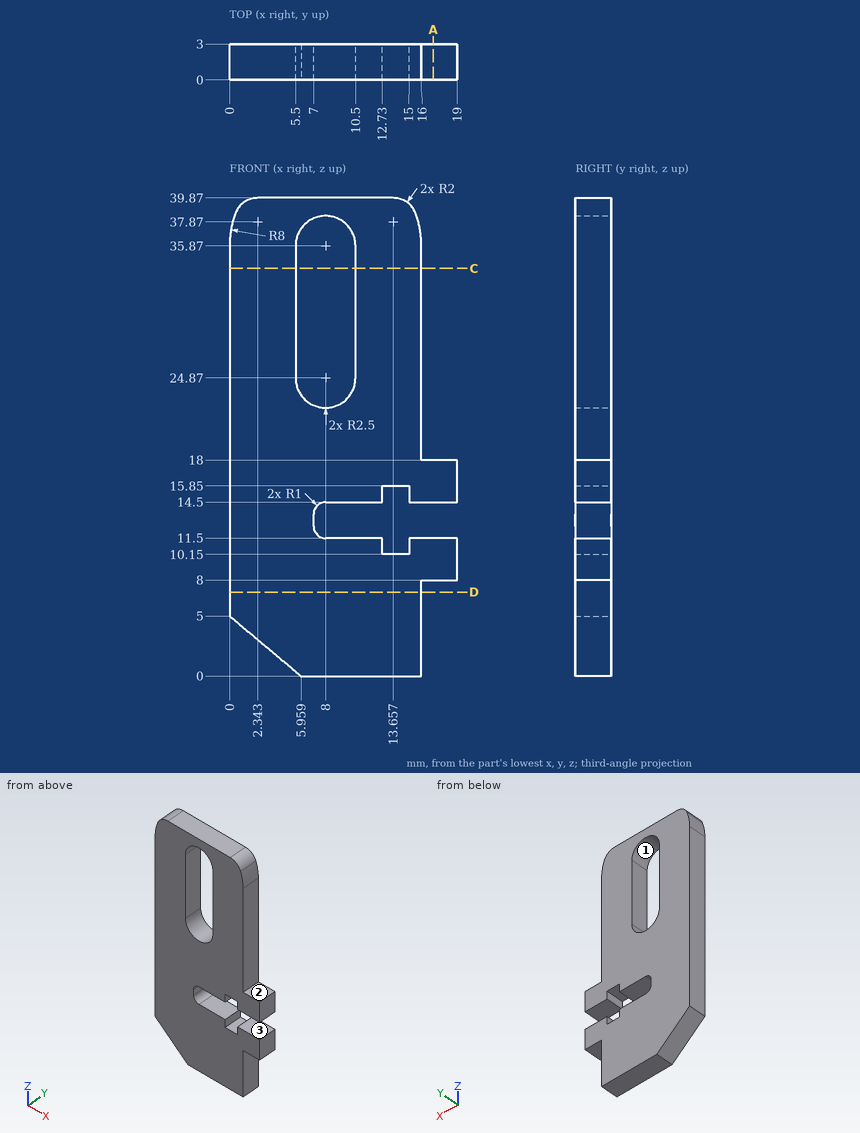
Part print with two shaded views. Sizes in mm from the minimum x, y, z corner. A direction names the side the tool comes from. Give positions to 0.01 mm unless a question says otherwise; leave off trailing zeros. Order: outer loops, then holes, each group sorted by start corner. A loop starts at its lowest first (then second) coordinate and runs counter-clockwise, first axis right, second up. Notation, with made-up numbers: M -4.5,82 L 19.5,82 A36 ccw 19.5,121 Z; hole C 87.25,51 d3. An arc over 180 degrees is marked long. Use one line per item in the form item = value.
1) Saw through at A-A (x = 17). Give the cut face in (y, z), plus the area to 3 significant figures.
Calculated:
outline = M 0,8 L 3,8 L 3,11.5 L 0,11.5 Z; M 0,14.5 L 3,14.5 L 3,18 L 0,18 Z
area = 21.0 mm2
2) Tool access for the marked faces 1, 2 and 3: list every direction of +Z, -Z, +X, -X, +Y, -Y with a clear straight run to the whole face (end or side of a thin tool).
Calculated:
face_1 = +Y, -Y
face_2 = +Z, +X, +Y, -Y
face_3 = +X, +Y, -Y
3) Saw through at C-C (z = 34). Give the cut face in (x, y), plus the area to 3 significant figures.
Calculated:
outline = M 0,0 L 5.5,0 L 5.5,3 L 0,3 Z; M 10.5,0 L 16,0 L 16,3 L 10.5,3 Z
area = 33.0 mm2
4) Probe probe 1 along Z at (x, y) = (13, 0.5); probe 2 along X at (y, z) = (2.45, 29); probe 3 along Z at (x, y) = (12.5, 2). List the from-to ranges inside material, lowest first.
Calculated:
probe_1 = 0 to 10.15, 15.85 to 39.87
probe_2 = 0 to 5.5, 10.5 to 16
probe_3 = 0 to 11.5, 14.5 to 39.87
5) Saw through at D-D (z = 7). Give the cut face in (x, y), plus the area to 3 significant figures.
Calculated:
outline = M 0,0 L 16,0 L 16,3 L 0,3 Z
area = 48.0 mm2
